Work out the finished part from the listing and answer in its coordinate system (mm). A direction names the side the tool comes from. Give positions to 0.01 mm unless a question says otherwise; leave off trailing zeros. Write each loop counter-clockwise with the first axis right and the second up, starting at its lowest first coordinate (ties: lowest second). Pieces come first, ordered by that corner, then holes. Notation, with made-up numbers: (-18.75, 11.25) - (37.25, 11.25) arc R8 ccw to (37.25, 16.25) - close; hole circle Ø9 at (43, 6.25). An arc over 180 degrees is marked (long way). Write item = value, one per line.
Autodesk Inventor part; units mm, degrees
ref_plane "YZ Plane" through (0, 0, 0) normal (1, 0, 0) x (0, 1, 0)
ref_plane "XZ Plane" through (0, 0, 0) normal (0, 1, 0) x (-1, 0, 0)
ref_plane "XY Plane" through (0, 0, 0) normal (0, 0, 1) x (1, 0, 0)
sketch "Sketch1" plane through (0, 0, 0) normal (0, 1, 0) x (-1, 0, 0)
  circle A0 centre (0, 0) radius 14.5
  circle A1 centre (0, 0) radius 10.5
  line L0 (14.5, 0) -> (7.5, 0)
  line L1 (-14.5, 0) -> (-7.5, 0)
  line L2 (7.5, -7.3485) -> (7.5, 7.3485)
  line L3 (-7.5, -7.3485) -> (-7.5, 7.3485)
  dimension "d0" = 29
  dimension "d1" = 21
  dimension "d2" = 7
  dimension "d3" = 7
extrude "Extrusion1" add sketch "Sketch1" along normal blind 4 contours L0 A1 L1 A0 | A0 L1 A1 L0 | L0 L2 A1 | A1 L2 L0 | L1 L3 A1 | A1 L3 L1
properties part number "LoadCellFitting"
1. Straight lines are drawn through the part: line 1 (Z direction, x = 10, y = 0.5); line 2 (Z direction, x = 5.25, y = 1.25); line 3 (X direction, y = 0.5, z = 3.5). For each, find the intervals that lie inside material, in ascending order.
Solution:
line_1 = -10.5 to 10.5
line_2 = -13.52 to -9.09, 9.09 to 13.52
line_3 = -14.07 to -7.5, 7.5 to 14.07
2. Find section D-D, the plane x = -9.5. Give the vertices of the cut face in (y, z).
Solution:
outline = (0, -10.95) - (4, -10.95) - (4, 10.95) - (0, 10.95) - close
3. Find section A-A, the plane x = 0. Give the vertices of the cut face in (y, z).
Solution:
outline = (0, -14.5) - (4, -14.5) - (4, -10.5) - (0, -10.5) - close; (0, 10.5) - (4, 10.5) - (4, 14.5) - (0, 14.5) - close
4. Given pin 1 (2 mm diameter, centred on y = 1.5, z = -4, fed in from +X); pin 2 (1 mm diameter, centred on x = 5, y = 1.5, fed in from +Z), each flat-ended and moving along its own axis, determine where each tip first touches the part or whether it passes through.
Solution:
pin_1 = 14.19
pin_2 = 13.78
5. Find section C-C, the plane y = 0.55. Give the vertices of the cut face in (x, z), then the cut area to 3 significant figures.
Solution:
outline = circle Ø29 at (0, 0); hole (-7.5, -7.35) arc R10.5 ccw to (7.5, -7.35) - (7.5, 7.35) arc R10.5 ccw to (-7.5, 7.35) - close
area = 375 mm^2
6. A tool of negligible diameter and unlimited length cuts with its end or side. For faces 4 (the cylindrical face through (0.1, 2, 10.5)), 5 (the flat face through (-9, 4, 0)), from which of +Z, -Z, +X, -X, +Y, -Y can it reach the whole face along a straight path? Write none if from no direction.
Solution:
face_4 = +Y, -Y
face_5 = +Z, -Z, +X, -X, +Y
7. Find section B-B, the plane z = 0. Give the vertices of the cut face in (x, y).
Solution:
outline = (-14.5, 0) - (-7.5, 0) - (-7.5, 4) - (-14.5, 4) - close; (7.5, 0) - (14.5, 0) - (14.5, 4) - (7.5, 4) - close
8. For a pull along X with two mould halves and no side action, classify faces 1 (the cylindrical face through (-0.1, 2, -10.5)), 2 (the cylindrical face through (-6.691, 1.972, 12.864)), 3 (the flat face through (-9, 0, 0)) as pulls with the +X half, pulls with the -X half, needs draft (parallel to the pull), parting line crosses it, or undercut.
Solution:
face_1 = undercut
face_2 = parting line crosses it
face_3 = needs draft
